Here's how the part is built. I have some questions about the finished solid (model axes, mm). Face numbers are marked on the shaded views. A direction names the side the tool comes from. Give positions to 0.01 mm unless a question says otherwise; leave off trailing zeros. Write each loop counter-clockwise with the first axis right and the second up, starting at its lowest first coordinate (ties: lowest second). Pieces come first, ordered by that corner, then holes. Notation, with made-up numbers: (28, 15) -> (36, 15) arc R11 ccw to (36, 20) -> close; hole circle Ø9 at (-23, 77). An arc over 180 degrees is marked (long way). Use CSV: the item, a comma, the result in double quotes. Start each with the question number.
(1) For pin 1 Ø0.8 at (x, z) = (0, -0.5) entering from +Y; pin 2 Ø2 at (y, z) = (-24.5, 1.5) entering from -X; pin 3 Ø2 at (x, y) = (-2, -39.5) entering from +Z, each with a flat end and sliding along its axis, tell me the tip position at first contact or that it passes through.
(2) I need wall thicknesses on L1, parallel to Z at x = -0.25, y = -88; L2, parallel to X at y = -79.5, z = -0.15; L3, parallel to Z at x = 0.1, y = -16. Which ranges of each line are inside material? Lowest first, please. Write a range as [from, to].
(3) Suppose I cut it at B-B on y = -12. List the corners of the cut face in (x, z) for me, plus the area to 3 significant figures.
(4) Which directions (+Z, -Z, +X, -X, +Y, -Y) give clear straight access to the entire face, cutting with the end or side of a thin tool? Please do the marked faces 1 and 2.
(5) Suppose I cut it at A-A on y = -36. List the corners of the cut face in (x, z) for me.
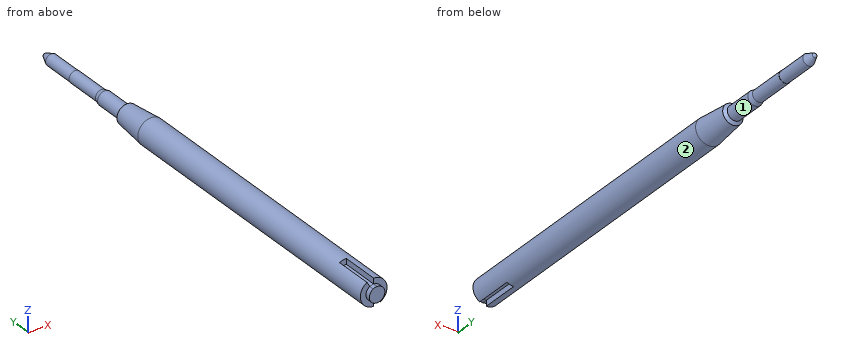
from build123d import *

# Parameters (mm, degrees)
SKIZZE2_W               = 3
SKIZZE2_H               = 9
SCHNITT_ROTATION1_ANGLE = 30


with BuildPart() as part:
    # Skizze1 → Rotation1 (revolve)
    with BuildSketch(Plane.XY, mode=Mode.PRIVATE) as rotation1_sk:
        with BuildLine():
            Line((1.25, -17.5), (1.5, -18.5))
            Line((1.5, -18.5), (1.5, -24.5))
            Line((1.5, -24.5), (2.1, -25))
            Line((2.1, -25), (2.75, -32))
            Line((2.75, -32), (2.75, -97))
            Line((2.75, -97), (1.6, -97))
            Line((1.6, -97), (1.6, -98))
            Line((1.6, -98), (0, -98))
            Line((0, -98), (0, -0.8))
            ThreePointArc((0, -0.8), (0.277350098, -0.883974853), (0.461538462, -1.107692308))
            Line((0.461538462, -1.107692308), (1.2, -2.88))
            Line((1.2, -2.88), (1.2, -9.8))
            Line((1.2, -9.8), (1.25, -9.8))
            Line((1.25, -9.8), (1.25, -17.5))
        make_face()
    revolve(rotation1_sk.sketch.rotate(Axis((0, 4.010416667, 0), (0, -1, 0)), 90), axis=Axis((0, 4.010416667, 0), (0, -1, 0)))

    # Skizze2 → Schnitt-Rotation1 (revolve, cut)
    with BuildSketch(Plane(origin=(0, 0, 0), x_dir=(0, 0, -1), z_dir=(1, 0, 0))):
        with Locations((-3.1, -93.5)):
            Rectangle(SKIZZE2_W, SKIZZE2_H)
        with Locations((3.1, -93.5)):
            Rectangle(SKIZZE2_W, SKIZZE2_H)
    revolve(axis=Axis((0, -78.967863002, 0), (0, -1, 0)), revolution_arc=SCHNITT_ROTATION1_ANGLE, mode=Mode.SUBTRACT)


solid = part.part
Geometry says:
1,pin 1,"y = -0.81"
1,pin 2,"x = -2"
1,pin 3,"z = 2.56"
2,L1,"[-2.74, 2.74]"
2,L2,"[-2.75, 2.75]"
2,L3,"[-1.25, 1.25]"
3,outline,"circle Ø2.5 at (0, 0)"
3,area,"4.91 mm²"
4,face 1,"+Y"
4,face 2,"+Y, -Y"
5,outline,"circle Ø5.5 at (0, 0)"
